from build123d import *

# Parameters (mm, degrees)
FILLET1_R    = 0.1
FILLET2_R    = 0.08
HEX_2_DEPTH  = 0.7
SCALE1_SCALE = 2.5


with BuildPart() as part:
    # BodySke → BaseBody (revolve)
    with BuildSketch(Plane.XY, mode=Mode.PRIVATE) as basebody_sk:
        Polygon((0, 0), (0, 1.5), (1.6, 1.5), (1.6, 0.8), (9.401, 0.8), (9.6, 0.601), (9.6, 0), align=None)
    revolve(basebody_sk.sketch.rotate(Axis((0, 0, 0), (1, 0, 0)), 90), axis=Axis((0, 0, 0), (1, 0, 0)))

    # Fillet1
    fillet1_edges = [part.edges().sort_by_distance(p)[0] for p in [
        (1.6, 0, -0.8),
    ]]
    fillet(fillet1_edges, radius=FILLET1_R)

    # Fillet2
    fillet2_edges = [part.edges().sort_by_distance(p)[0] for p in [
        (0, 0, -1.5),
    ]]
    fillet(fillet2_edges, radius=FILLET2_R)

    # HexSke → Hex 2 (cut)
    with BuildSketch(Plane(origin=(0, 0, 0), x_dir=(0, 0, -1), z_dir=(1, 0, 0))):
        Polygon((0, 0.866025404), (-0.75, 0.433012702), (-0.75, -0.433012702), (0, -0.866025404), (0.75, -0.433012702), (0.75, 0.433012702), align=None)
    extrude(amount=HEX_2_DEPTH, mode=Mode.SUBTRACT)

    # Hex-PreBroachSke → Hex-PreBroach (revolve, cut)
    with BuildSketch(Plane.XY, mode=Mode.PRIVATE) as hex_prebroach_sk:
        Polygon((0, 0), (0, 0.75), (0.7, 0.75), (1.133012702, 0), align=None)
    revolve(hex_prebroach_sk.sketch.rotate(Axis((0, 0, 0), (1, 0, 0)), 270), axis=Axis((0, 0, 0), (1, 0, 0)), mode=Mode.SUBTRACT)


with BuildPart() as part_1:
    # Scale1: scaled about (3.799750462, 0, 0)
    add(part.part.scale(SCALE1_SCALE).moved(Location((-5.699625693, 0, 0))))


solid = part_1.part
Input: part model. Units: mm. Frame: model coordinates. A direction names the side the tool comes from. Give positions to 0.01 mm unless a question says otherwise; leave off trailing zeros. Order: outer loops, then holes, each group sorted by start corner. A loop starts at its lowest first (then second) coordinate and runs counter-clockwise, first axis right, second up.
Q1. Draft query along Z for faces 4 (the cylindrical face through (-3.57, -3.16, 2.02)), 5 (the flat face through (-5, 0, -1.875)), 6 (the flat face through (-1.7, 2, 2)), 7 (the flat face through (-4.837, 1.631, 0.924)). Return one class per face: +Z half, -Z half, draft (parallel to the pull), parting line (faces both ways), or undercut.
Checked values:
face 4: parting line
face 5: undercut
face 6: draft
face 7: undercut
Q2. Ray query, probe 1 along X at (y, z) = (2.75, 1.25); probe 2 along Y at (x, z) = (-4.5, -3.25); probe 3 along Z at (x, y) = (10.25, 0.5). Return the intervals inside material, ascending.
Checked values:
probe 1: x = -5.7 to -1.7
probe 2: y = -1.87 to 1.87
probe 3: z = -1.94 to 1.94
Q3. Set-up query: faces 1 (the cylindrical face through (8, 2, 0)), 2 (the flat face through (-5.7, 2, -2)), 3 (the flat face through (-4.837, -1.631, -0.924)). Return all of +Z, -Z, +X, -X, +Y, -Y with unobstructed straight access to the full face (end or side cutting, diameter ignored); none if empty.
Checked values:
face 1: +X
face 2: +Z, -Z, -X, +Y, -Y
face 3: -X
Q4. Section A-A on x = 2.75. Output: boundary loops of the cut face in (y, z), and give its area (3 significant figures).
Checked values:
outline: circle Ø4 at (0, 0)
area: 12.6 mm2
